Read the model definition and answer for the solid it produces. Units are mm, in the model's axes. A direction names the side the tool comes from. Round coordinates to 2 decimals unless told otherwise and drop trailing zeros. Loops run counter-clockwise (first coordinate to the right, second up) from the corner with the lowest first, then second, coordinate; pieces in that order, holes last. Notation, with made-up numbers: M 50.5,-7 L 59.5,-7 A17 cw 59.5,4 Z; hole C 68.25,-5.5 d11. An arc over 180 degrees is marked long. Answer as CSV lines item,"result".
Autodesk Inventor part; units mm, degrees
ref_plane "YZ Plane" through (0, 0, 0) normal (1, 0, 0) x (0, 1, 0)
ref_plane "XZ Plane" through (0, 0, 0) normal (0, 1, 0) x (-1, 0, 0)
ref_plane "XY Plane" through (0, 0, 0) normal (0, 0, 1) x (1, 0, 0)
sketch "Sketch1" plane through (0, 0, 0) normal (0, 1, 0) x (-1, 0, 0)
  line L0 (-33.65, -40) -> (33.65, -40)
  line L1 (40, -33.65) -> (40, 33.65)
  line L2 (33.65, 40) -> (-33.65, 40)
  line L3 (-40, 33.65) -> (-40, -33.65)
  line L4 (-40, -40) -> (40, 40) construction
  line L5 (40, -40) -> (-40, 40) construction
  arc A0 (40, 33.65) -> (33.65, 40) centre (33.65, 33.65) ccw
  arc A1 (-33.65, 40) -> (-40, 33.65) centre (-33.65, 33.65) ccw
  arc A2 (-40, -33.65) -> (-33.65, -40) centre (-33.65, -33.65) ccw
  arc A3 (33.65, -40) -> (40, -33.65) centre (33.65, -33.65) ccw
  point P0 (0, 0)
  dimension "d0" = 80
  dimension "d1" = 80
  dimension "d2" = 6.35
extrude "Extrusion1" add sketch "Sketch1" along normal blind 25.4
shell "Shell1" thickness 1.7 removed faces 1 at (-11.2167, 25.4, 9.1)
fillet "Fillet1" radius 1.27 8 edges at (-38.1401, 0, -38.1401) (-40, 0, 0) (-38.1401, 0, 38.1401) (0, 0, 40) (38.1401, 0, 38.1401) (40, 0, 0) (38.1401, 0, -38.1401) (0, 0, -40)
sketch "Sketch2" plane through (-33.65, 1.7, 38.3) normal (0, 1, 0) x (1, 0, 0)
  arc A0 (-4.65, 4.65) -> (0, 0) centre (0, 4.65) ccw
  circle A1 centre (0, 4.65) radius 3.175
  circle A2 centre (0, 4.65) radius 1.2
  point P0 (33.65, 38.3)
  dimension "d7" = 6.35
  dimension "d8" = 2.4
extrude "Extrusion2" add sketch "Sketch2" along normal up to surface (23.7 mm away)
mirror "Mirror1" about plane through (0, 0, 0) normal (1, 0, 0) of "Extrusion2"
mirror "Mirror2" about plane through (0, 0, 0) normal (0, 0, 1) of "Extrusion2", "Mirror1"
sketch "Sketch3" plane through (-40, 25.4, -33.65) normal (-1, 0, 0) x (0, 0, 1)
  line L0 (0, 0) -> (67.3, 0)
  line L1 (11.43, 0) -> (25.43, 0)
  line L2 (25.43, 0) -> (25.43, -21.59)
  line L3 (25.43, -21.59) -> (11.43, -21.59)
  line L4 (11.43, -21.59) -> (11.43, 0)
  line L5 (-6.35, -24.13) -> (-6.35, 0)
  point P0 (33.65, -25.4)
  dimension "d11" = 14
  dimension "d12" = 21.59
  dimension "d13" = 17.78
extrude "Extrusion3" cut sketch "Sketch3" against normal blind 25.4
properties part number "Arduino_case_bottom_JC_Rev1"
1) A tool of negligible diameter and unlimited length cuts with its end or side. For faces 5 (the cylindrical face through (35.99, 13.384, -35.796)), 6 (the flat face through (1, 0, 1)), from which of +Z, -Z, +X, -X, +Y, -Y can it reach the whole face along a straight path? Write none if from no direction.
Evaluation:
face 5,"+Y"
face 6,"+Z, -Z, +X, -X, -Y"
2) Find section B-B, the plane z = 29.5. Give the vertices of the cut face in (x, y), then the cut area to 3 significant figures.
Evaluation:
outline,"M -40,1.27 A1.27 ccw -38.73,0 L 38.73,0 A1.27 ccw 40,1.27 L 40,25.4 L 38.3,25.4 L 38.3,1.7 L -38.3,1.7 L -38.3,25.4 L -40,25.4 Z"
area,"216 mm^2"
3) Find section A-A, the plane y = 11.5. Count the separate pieces of the cut face and the enclosed holes in it, then the cut area to 3 significant figures.
Evaluation:
separate pieces,"5"
enclosed holes,"4"
area,"601 mm^2"
4) Each of these flat-tipped pins is pushed along its axis until it touches: P1, Ø0.5, axis at x = -39, y = 14, coming from the -Z side; P2, Ø1.9, axis at x = -33.5, z = -33.5, coming from the +Y side; P3, Ø1.4, axis at x = -39.5, y = 17.5, coming from the +Z side. Where does it stop, or does it pass through?
Evaluation:
P1,"stops at z = -37.43"
P2,"stops at y = 1.7"
P3,"stops at z = 37.36"
5) Straight lines are drawn through the part: line 1 (X direction, y = 22, z = -33.5); line 2 (Z direction, x = 33.65, y = 15.75) (3 decimals); line 3 (X direction, y = 24.25, z = -25.5). For each, find the intervals that lie inside material, in ascending order.
Evaluation:
line 1,"x = -40 to -38.3, -36.82 to -34.84, -32.46 to -30.48, 30.48 to 32.46, 34.84 to 36.82, 38.3 to 40"
line 2,"z = -40 to -38.3, -36.825 to -34.85, -32.45 to -30.475, 30.475 to 32.45, 34.85 to 36.825, 38.3 to 40"
line 3,"x = -40 to -38.3, 38.3 to 40"
6) Determine the mould class of faces 1 (the flat face through (-34, 25.4, 35)), 2 (the flat face through (-40, 13, 0)), 3 (the cylindrical face through (36.902, 13.384, -36.974)), 4 (the cylindrical face through (-33.096, 13.384, 32.585)) for opening direction X: released by +X, released by -X, zero draft, split by the parting line, or undercut.
Evaluation:
face 1,"zero draft"
face 2,"released by -X"
face 3,"undercut"
face 4,"undercut"
7) Find section C-C, the plane x = 29.5. Give the vertices of the cut face in (y, z), then the cut area to 3 significant figures.
Evaluation:
outline,"M 0,-38.73 A1.27 ccw 1.27,-40 L 25.4,-40 L 25.4,-38.3 L 1.7,-38.3 L 1.7,38.3 L 25.4,38.3 L 25.4,40 L 1.27,40 A1.27 ccw 0,38.73 Z"
area,"216 mm^2"
8) Find section D-D, the plane z = -31.5. Give the vertices of the cut face in (x, y), then the cut area to 3 significant figures.
Evaluation:
outline,"M -40,1.27 A1.27 ccw -38.73,0 L 38.73,0 A1.27 ccw 40,1.27 L 40,25.4 L 38.3,25.4 L 38.3,1.7 L 35.99,1.7 L 35.99,25.4 L 31.31,25.4 L 31.31,1.7 L -31.31,1.7 L -31.31,25.4 L -35.99,25.4 L -35.99,1.7 L -38.3,1.7 L -38.3,25.4 L -40,25.4 Z"
area,"437 mm^2"
